from build123d import *

# Parameters (mm, degrees)
F0_R     = 12.1654817783
F0_R_2   = 12.3094418461
F1_DEPTH = 254


with BuildPart() as f1:
    # F0 (on Front) → F1 (new body)
    with BuildSketch(Plane.XZ):
        with BuildLine():
            Line((-244.6754564072, -95.9572500223), (-248.3565956354, -94.854135785))
            Line((-248.3565956354, -94.854135785), (-248.3565956354, -127.5566222325))
            ThreePointArc((-248.3565956354, -127.5566222325), (-213.8078944202, -125.8910654203), (-179.4121861458, -122.2411219335))
            Line((-179.4121861458, -122.2411219335), (-179.4121861458, -58.1807047129))
            Line((-179.4121861458, -58.1807047129), (-217.1610821121, -70.0124311765))
            Line((-217.1610821121, -70.0124311765), (-244.6754564072, -95.9572500223))
        make_face()
        with BuildLine():
            Line((-248.3565956354, -127.5566222325), (-248.3565956354, -94.854135785))
            Line((-248.3565956354, -94.854135785), (-290.3897309912, -82.2582117584))
            Line((-290.3897309912, -82.2582117584), (-301.3831531393, -35.8189695212))
            Line((-301.3831531393, -35.8189695212), (-266.6623007034, -3.0787655479))
            Line((-266.6623007034, -3.0787655479), (-220.9480261194, -16.7778038117))
            Line((-220.9480261194, -16.7778038117), (-209.9546039713, -63.2170460489))
            Line((-209.9546039713, -63.2170460489), (-217.1610821121, -70.0124311765))
            Line((-217.1610821121, -70.0124311765), (-179.4121861458, -58.1807047129))
            Line((-179.4121861458, -58.1807047129), (-179.4121861458, -122.2411219335))
            ThreePointArc((-179.4121861458, -122.2411219335), (-157.6679238797, -118.8925887902), (-136.0607594252, -114.7506013513))
            ThreePointArc((-136.0607594252, -114.7506013513), (-139.0216639455, -70.9358153589), (-96.8521743572, -58.6787123162))
            ThreePointArc((-96.8521743572, -58.6787123162), (-38.8407590079, 4.8396231382), (18.5831978775, -59.210298215))
            ThreePointArc((18.5831978775, -59.210298215), (-409.1140131264, 1055.7782487651), (-248.3565956354, -127.5566222325))
        make_face()
        with Locations((-160.0868552923, 12.0240524411)):
            Circle(F0_R, mode=Mode.SUBTRACT)
        with Locations((-132.9269260168, 20.9090542048)):
            Circle(F0_R_2, mode=Mode.SUBTRACT)
        with BuildLine():
            ThreePointArc((-179.4121861458, -122.2411219335), (-213.8078944202, -125.8910654203), (-248.3565956354, -127.5566222325))
            Line((-248.3565956354, -127.5566222325), (-248.3565956354, -167.3867851496))
            Line((-248.3565956354, -167.3867851496), (-179.4121861458, -147.1127271652))
            Line((-179.4121861458, -147.1127271652), (-179.4121861458, -122.2411219335))
        make_face()
        with BuildLine():
            ThreePointArc((-75.2215410202, -98.5602818592), (-27.4853011776, -80.873117917), (18.5831978775, -59.210298215))
            ThreePointArc((18.5831978775, -59.210298215), (-38.8407590079, 4.8396231382), (-96.8521743572, -58.6787123162))
            ThreePointArc((-96.8521743572, -58.6787123162), (-79.3970992955, -74.572736982), (-75.9955495596, -97.9335829616))
            ThreePointArc((-75.9955495596, -97.9335829616), (-75.60989028, -98.2485935492), (-75.2215410202, -98.5602818592))
        make_face()
        with BuildLine():
            ThreePointArc((-75.2215410202, -98.5602818592), (-16.6690404085, -106.6575382222), (18.5831978775, -59.210298215))
            ThreePointArc((18.5831978775, -59.210298215), (-27.4853011776, -80.873117917), (-75.2215410202, -98.5602818592))
        make_face()
    extrude(amount=F1_DEPTH)


solid = f1.part
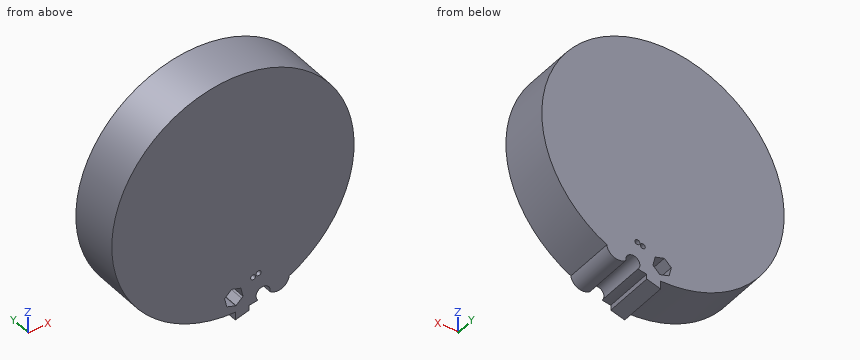
Verification items for the finished model (mm, model axes). Give positions to 0.01 mm unless a question says otherwise; leave off trailing zeros. Write each loop counter-clockwise with the first axis right and the second up, starting at its lowest first coordinate (ties: lowest second). Pieces come first, ordered by that corner, then holes.
(1) Material ranges on line 1 (X direction, y = -126, z = 8.5); line 2 (X direction, y = -38, z = -37.5); line 3 (X direction, y = -194.5, z = 490), recorded low to high.
(2) Cross-section at C-C (z = 794). Enter the section's corners in (x, y), plus the area to 3 significant figures.
(3) Gauge pin test, flat ends, axial feed: pin 1 (12 mm diameter, centred on y = -96.5, z = -142.5, fed in from -X); pin 2 (6 mm diameter, centred on y = -167.5, z = 706.5, fed in from +X); pin 3 (1.5 mm diameter, centred on y = -48.5, z = 236, fed in from -X). Record the tip position at first contact, or that the pin passes through.
(4) Cross-section at A-A (y = -223). Enter the section's corners in (x, z), plus the area to 3 significant figures.
(5) Cross-section at B-B (x = -376.5). Enter the section's corners in (y, z).
Worked out:
1. line 1: x = -641.02 to -171.73, -148.44 to 120.99
1. line 2: x = -576.68 to -300.99, -216.04 to 56.65
1. line 3: x = -860.9 to 340.87
2. outline: (-768.53, -254) - (248.5, -254) - (248.5, 0) - (-768.53, 0) - close
2. area: 258,000 mm2
3. pin 1: stops at x = -248.36
3. pin 2: stops at x = 295.34
3. pin 3: stops at x = -812.57
4. outline: (-248.36, -167.39) - (-179.41, -147.11) - (-179.41, -122.24) arc R601.12 ccw to (-136.06, -114.75) arc R35.02 cw (long way) to (-76, -97.93) arc R58.01 ccw to (18.58, -59.21) arc R601.12 ccw (long way) to (-248.36, -127.56) - close; hole (-301.38, -35.82) - (-290.39, -82.26) - (-244.68, -95.96) - (-209.95, -63.22) - (-220.95, -16.78) - (-266.66, -3.08) - close; hole circle Ø24.33 at (-160.09, 12.02); hole circle Ø24.62 at (-132.93, 20.91)
4. area: 1,130,000 mm2
5. outline: (-254, -116.28) - (0, -116.28) - (0, 1063.17) - (-254, 1063.17) - close
